from build123d import *

# Parameters (mm, degrees)
BOSS_EXTRUDE1_DEPTH      = 6
MOUNT_SCREW_HOLES_REACH  = 65.711
SKETCH12_R               = 1.5
GEAR_START               = 6
SKETCH13_R               = 4
GEAR_SHAFT_DEPTH         = 8
SKETCH14_R               = 1.5
GEAR_SCREW_HOLE_DEPTH    = 65.954522552
SKETCH15_R               = 0.975
SERVO_SCREW_CUTOUT_DEPTH = 65.954522552
FILLET1_R                = 4


with BuildPart() as part:
    # body → Boss-Extrude1 (new body)
    with BuildSketch(Plane.XY):
        with BuildLine():
            Line((-24.5, 4.5), (24.5, 4.5))
            Line((24.5, 4.5), (24.5, -31.14142872))
            ThreePointArc((24.5, -31.14142872), (29.953423421, -39.424986813), (21.650045301, -44.848184531))
            Line((21.650045301, -44.848184531), (-44.7, -30.8))
            Line((-44.7, -30.8), (-44.7, -14.6))
            Line((-44.7, -14.6), (-40, -14.6))
            Line((-40, -14.6), (-40, -26.8))
            Line((-40, -26.8), (-17, -26.8))
            Line((-17, -26.8), (-17, -4.5))
            Line((-17, -4.5), (-24.5, -4.5))
            Line((-24.5, -4.5), (-24.5, 4.5))
        make_face()
        with BuildLine():
            Line((-12.3, 0.5), (14.5, 0.5))
            Line((14.5, 0.5), (14.5, -5.5))
            Line((14.5, -5.5), (20.5, -5.5))
            Line((20.5, -5.5), (20.5, -31.500769276))
            ThreePointArc((20.5, -31.500769276), (16.884558972, -34.780016642), (16.291201999, -39.624890698))
            Line((16.291201999, -39.624890698), (-12.3, -33.571323141))
            Line((-12.3, -33.571323141), (-12.3, 0.5))
        make_face(mode=Mode.SUBTRACT)
    extrude(amount=BOSS_EXTRUDE1_DEPTH)

    # Sketch12 → mount screw holes (cut, up to next)
    with BuildSketch(Plane.XY, mode=Mode.PRIVATE) as mount_screw_holes_sk1:
        with Locations(Location((20, 0, 0), (0, 0, 180))):
            Circle(SKETCH12_R)
    mount_screw_holes_tool1 = extrude(mount_screw_holes_sk1.sketch, amount=MOUNT_SCREW_HOLES_REACH, mode=Mode.PRIVATE) & part.part
    # Sketch12 → mount screw holes (cut, up to next)
    with BuildSketch(Plane.XY, mode=Mode.PRIVATE) as mount_screw_holes_sk2:
        with Locations(Location((-20, 0, 0), (0, 0, 180))):
            Circle(SKETCH12_R)
    mount_screw_holes_tool2 = extrude(mount_screw_holes_sk2.sketch, amount=MOUNT_SCREW_HOLES_REACH, mode=Mode.PRIVATE) & part.part
    add(mount_screw_holes_tool1.solids().sort_by_distance((20, 0, 0))[0], mode=Mode.SUBTRACT)
    add(mount_screw_holes_tool2.solids().sort_by_distance((-20, 0, 0))[0], mode=Mode.SUBTRACT)

    # Sketch13 → gear shaft (add)
    with BuildSketch(Plane.XY.offset(GEAR_START)):
        with Locations((23.1, -38)):
            Circle(SKETCH13_R)
    extrude(amount=GEAR_SHAFT_DEPTH)

    # Sketch14 → gear screw hole (cut, through all)
    with BuildSketch(Plane.XY):
        with Locations((23.1, -38)):
            Circle(SKETCH14_R)
    extrude(amount=GEAR_SCREW_HOLE_DEPTH, mode=Mode.SUBTRACT)

    # Sketch15 → servo screw cutout (cut, through all)
    with BuildSketch(Plane.XY):
        with Locations((-14.6, -20.7)):
            Circle(SKETCH15_R)
        with Locations((-42.4, -20.7)):
            Circle(SKETCH15_R)
    extrude(amount=SERVO_SCREW_CUTOUT_DEPTH, mode=Mode.SUBTRACT)

    # Fillet1
    fillet1_edges = [part.edges().sort_by_distance(p)[0] for p in [
        (-24.5, -4.5, 3),
        (-24.5, 4.5, 3),
        (24.5, 4.5, 3),
        (24.5, -31.14142872, 3),
        (-44.7, -30.8, 3),
        (-44.7, -14.6, 3),
        (14.5, -5.5, 3),
        (-12.3, 0.5, 3),
        (-12.3, -33.571323141, 3),
        (16.291201999, -39.624890698, 3),
        (20.5, -31.500769276, 3),
    ]]
    fillet(fillet1_edges, radius=FILLET1_R)


solid = part.part
Model file for the job. Use its own axes, mm. A direction names the side the tool comes from. Give positions to 0.01 mm unless a question says otherwise; leave off trailing zeros. Order: outer loops, then holes, each group sorted by start corner. A loop starts at its lowest first (then second) coordinate and runs counter-clockwise, first axis right, second up. Notation, with made-up numbers: M 44,51.25 L 50,51.25 A23 cw 50,64.25 Z; hole C 17,38 d8. An arc over 180 degrees is marked long. Write item = value, one per line.
Q1. Flat gauge pins, fed straight in: pin 1 (0.8 mm diameter, centred on x = -40, z = 2, fed in from +Y); pin 2 (4 mm diameter, centred on x = 13.5, z = 6.5, fed in from -Y); pin 3 (8 mm diameter, centred on y = -8.5, z = 11, fed in from -X); pin 4 (1.6 mm diameter, centred on y = -1, z = 3.5, fed in from -X). Where does each tip first touch, or does it go through?
Derived:
pin_1 = -14.6
pin_2 = -43.53
pin_3 = through
pin_4 = -24.5
Q2. Cut at A-A, the plane x = -42.4. List the corners of the cut face in (y, z) (3 decimals), then the cut area to 3 significant figures.
Derived:
outline = M -31.179,0 L -21.675,0 L -21.675,6 L -31.179,6 Z; M -19.725,0 L -14.979,0 L -14.979,6 L -19.725,6 Z
area = 85.5 mm2
Q3. Cut at B-B, the plane y = -8. List the corners of the cut face in (x, z).
Derived:
outline = M -17,0 L -12.3,0 L -12.3,6 L -17,6 Z; M 20.5,0 L 24.5,0 L 24.5,6 L 20.5,6 Z
Q4. Tool access for faces 1 (the cylindrical face through (-11.097, -0.641, 3.042)), 2 (the cylindrical face through (25.25, -34.627, 9.944)), 3 (the flat face through (-19, -4.5, 3)), 4 (the cylindrical face through (-43.78, -30.11, 3.04)): list every direction of +Z, -Z, +X, -X, +Y, -Y with a clear straight run to the whole face (end or side of a thin tool).
Derived:
face_1 = +Z, -Z
face_2 = +Z
face_3 = +Z, -Z, -X
face_4 = +Z, -Z, -X, -Y
Q5. Two-plate mould, pull along Y, no slides. Class faces 5 (the flat face through (24.5, -14, 3)), 6 (the cylindrical face through (21.5, -0.07, 2.96)), 7 (the cylindrical face through (29.697, -40.341, 2.958)): pulls with the +Y half, pulls with the -Y half, needs draft (parallel to the pull), parting line crosses it, or undercut.
Derived:
face_5 = needs draft
face_6 = undercut
face_7 = parting line crosses it
Q6. Drill centre lines: line 1 (X direction, y = -19, z = 5); line 2 (X direction, y = -20.7, z = 2.5) (3 decimals); line 3 (X direction, y = -8, z = 3). Where is each one in solid material? Low to high. Write a range as [from, to].
Derived:
line_1 = [-44.7, -40], [-17, -12.3], [20.5, 24.5]
line_2 = [-44.7, -43.375], [-41.425, -40], [-17, -15.575], [-13.625, -12.3], [20.5, 24.5]
line_3 = [-17, -12.3], [20.5, 24.5]
Q7. Cut at C-C, the plane z = 4.75. Count the separate pieces of the cut face and the enclosed holes in it, then the cut area to 3 significant figures.
Derived:
separate_pieces = 1
enclosed_holes = 6
area = 1,060 mm2
Q8. Cut at D-D, the plane x = 22.5. List the corners of the cut face in (y, z), then the cut area to 3 significant figures.
Derived:
outline = M -44.97,0 L -39.37,0 L -39.37,14 L -41.95,14 L -41.95,6 L -44.97,6 Z; M -36.63,0 L 3.96,0 L 3.96,6 L -34.05,6 L -34.05,14 L -36.63,14 Z
area = 318 mm2
